Build history of the part. All positions in model axes, mm. Face numbers are marked on the shaded views. A direction names the side the tool comes from. Round coordinates to 2 decimals unless told otherwise and drop trailing zeros. Write each loop counter-clockwise with the first axis right and the second up, starting at its lowest first coordinate (ties: lowest second). Pieces come first, ordered by that corner, then holes. Notation, with made-up numbers: M 87.5,53.25 L 94.5,53.25 A9 ccw 94.5,64.25 Z; hole C -36.5,14 d10. An arc over 180 degrees is marked long. Use a Markdown table: item, result.
from build123d import *

# Parameters (mm, degrees)
F0_W         = 75
F0_H         = 75
F1_DEPTH     = 45
F2_T         = -2.5
F4_T1_DEPTH  = 49.5
F4_T3_DEPTH  = 69
F4_T5_DEPTH  = 69
F4_S9_W      = 3
F4_S9_H      = 3
F4_T10_DEPTH = 3
F4_S15_W     = 3
F4_S15_H     = 3
F4_T16_DEPTH = 3
F4_S21_W     = 3
F4_S21_H     = 3
F4_T22_DEPTH = 3
F4_S27_W     = 3
F4_S27_H     = 3
F4_T28_DEPTH = 3


# Not quite as in the source:
# - a fillet or chamfer that OpenCascade refuses, or shapes differently, is made with other operations: its cross-section is extruded or revolved along the edge and cut away or added
# - a feature of the source that left no trace in its solid (it failed there, or was rolled back) is left out


with BuildPart() as f1:
    # F0 (on Front) → F1 (new body)
    with BuildSketch(Plane.XZ):
        Rectangle(F0_W, F0_H)
    extrude(amount=F1_DEPTH)

    # F2
    f2_openings = [f1.faces().sort_by_distance(p)[0] for p in [
        (0, -45, 0),
    ]]
    offset(amount=F2_T, openings=f2_openings)

    # F4: fillet of radius 3 on 8 edges, made by hand

    # F4_s2 → F4_t1 (cut)
    with BuildSketch(Plane.XZ.offset(-7.5)):
        with BuildLine():
            ThreePointArc((-34.5, 37.5), (-36.6213203436, 36.6213203436), (-37.5, 34.5))
            Line((-37.5, 34.5), (-37.5, 37.5))
            Line((-37.5, 37.5), (-34.5, 37.5))
        make_face()
        with BuildLine():
            ThreePointArc((-34.5, -37.5), (-36.6213203436, -36.6213203436), (-37.5, -34.5))
            Line((-37.5, -34.5), (-37.5, -37.5))
            Line((-37.5, -37.5), (-34.5, -37.5))
        make_face()
        with BuildLine():
            ThreePointArc((34.5, -37.5), (36.6213203436, -36.6213203436), (37.5, -34.5))
            Line((37.5, -34.5), (37.5, -37.5))
            Line((37.5, -37.5), (34.5, -37.5))
        make_face()
        with BuildLine():
            ThreePointArc((37.5, 34.5), (36.6213203436, 36.6213203436), (34.5, 37.5))
            Line((34.5, 37.5), (37.5, 37.5))
            Line((37.5, 37.5), (37.5, 34.5))
        make_face()
    extrude(amount=F4_T1_DEPTH, mode=Mode.SUBTRACT)

    # F4_s4 → F4_t3 (cut)
    with BuildSketch(Plane.YZ.offset(-34.5)):
        with BuildLine():
            ThreePointArc((-42, -37.5), (-44.1213203436, -36.6213203436), (-45, -34.5))
            Line((-45, -34.5), (-45, -37.5))
            Line((-45, -37.5), (-42, -37.5))
        make_face()
        with BuildLine():
            ThreePointArc((-42, 37.5), (-44.1213203436, 36.6213203436), (-45, 34.5))
            Line((-45, 34.5), (-45, 37.5))
            Line((-45, 37.5), (-42, 37.5))
        make_face()
    extrude(amount=F4_T3_DEPTH, mode=Mode.SUBTRACT)

    # F4_s6 → F4_t5 (cut)
    with BuildSketch(Plane.XY.offset(-34.5)):
        with BuildLine():
            ThreePointArc((37.5, -42), (36.6213203436, -44.1213203436), (34.5, -45))
            Line((34.5, -45), (37.5, -45))
            Line((37.5, -45), (37.5, -42))
        make_face()
        with BuildLine():
            ThreePointArc((-37.5, -42), (-36.6213203436, -44.1213203436), (-34.5, -45))
            Line((-34.5, -45), (-37.5, -45))
            Line((-37.5, -45), (-37.5, -42))
        make_face()
    extrude(amount=F4_T5_DEPTH, mode=Mode.SUBTRACT)


with BuildPart() as f4_tool8:
    # F4_s9 → F4_t10 (new body)
    with BuildSketch(Plane.XY.offset(34.5)):
        with Locations((-36, -43.5)):
            Rectangle(F4_S9_W, F4_S9_H)
    extrude(amount=F4_T10_DEPTH)

    # F4_s11 → F4_t12 (revolve, cut)
    with BuildSketch(Plane(origin=(-34.5, -42, 34.5), x_dir=(0.7071067812, 0.7071067812, 0), z_dir=(0.7071067812, -0.7071067812, 0))):
        with BuildLine():
            ThreePointArc((0, -3), (3, 0), (0, 3))
            Line((0, 3), (0, -3))
        make_face()
    revolve(axis=Axis((-34.5, -42, 34.5), (0, 0, 1)), mode=Mode.SUBTRACT)


with BuildPart() as f1_1:
    add(f1.part)

    # F4_t7: cut F4_tool8
    add(f4_tool8.part, mode=Mode.SUBTRACT)


with BuildPart() as f4_tool14:
    # F4_s15 → F4_t16 (new body)
    with BuildSketch(Plane.XY.offset(-34.5)):
        with Locations((-36, -43.5)):
            Rectangle(F4_S15_W, F4_S15_H)
    extrude(amount=-F4_T16_DEPTH)

    # F4_s17 → F4_t18 (revolve, cut)
    with BuildSketch(Plane(origin=(-34.5, -42, -34.5), x_dir=(0.7071067812, 0.7071067812, 0), z_dir=(-0.7071067812, 0.7071067812, 0))):
        with BuildLine():
            ThreePointArc((0, -3), (3, 0), (0, 3))
            Line((0, 3), (0, -3))
        make_face()
    revolve(axis=Axis((-34.5, -42, -34.5), (0, 0, -1)), mode=Mode.SUBTRACT)


with BuildPart() as f1_2:
    add(f1_1.part)

    # F4_t13: cut F4_tool14
    add(f4_tool14.part, mode=Mode.SUBTRACT)


with BuildPart() as f4_tool20:
    # F4_s21 → F4_t22 (new body)
    with BuildSketch(Plane.XY.offset(-34.5)):
        with Locations((36, -43.5)):
            Rectangle(F4_S21_W, F4_S21_H)
    extrude(amount=-F4_T22_DEPTH)

    # F4_s23 → F4_t24 (revolve, cut)
    with BuildSketch(Plane(origin=(34.5, -42, -34.5), x_dir=(-0.7071067812, 0.7071067812, 0), z_dir=(-0.7071067812, -0.7071067812, 0))):
        with BuildLine():
            ThreePointArc((0, -3), (3, 0), (0, 3))
            Line((0, 3), (0, -3))
        make_face()
    revolve(axis=Axis((34.5, -42, -34.5), (0, 0, -1)), mode=Mode.SUBTRACT)


with BuildPart() as f1_3:
    add(f1_2.part)

    # F4_t19: cut F4_tool20
    add(f4_tool20.part, mode=Mode.SUBTRACT)


with BuildPart() as f4_tool26:
    # F4_s27 → F4_t28 (new body)
    with BuildSketch(Plane.YZ.offset(34.5)):
        with Locations((-43.5, 36)):
            Rectangle(F4_S27_W, F4_S27_H)
    extrude(amount=F4_T28_DEPTH)

    # F4_s29 → F4_t30 (revolve, cut)
    with BuildSketch(Plane(origin=(34.5, -42, 34.5), x_dir=(0, 0.7071067812, -0.7071067812), z_dir=(0, -0.7071067812, -0.7071067812))):
        with BuildLine():
            ThreePointArc((0, -3), (3, 0), (0, 3))
            Line((0, 3), (0, -3))
        make_face()
    revolve(axis=Axis((34.5, -42, 34.5), (1, 0, 0)), mode=Mode.SUBTRACT)


with BuildPart() as f1_4:
    add(f1_3.part)

    # F4_t25: cut F4_tool26
    add(f4_tool26.part, mode=Mode.SUBTRACT)


solid = f1_4.part
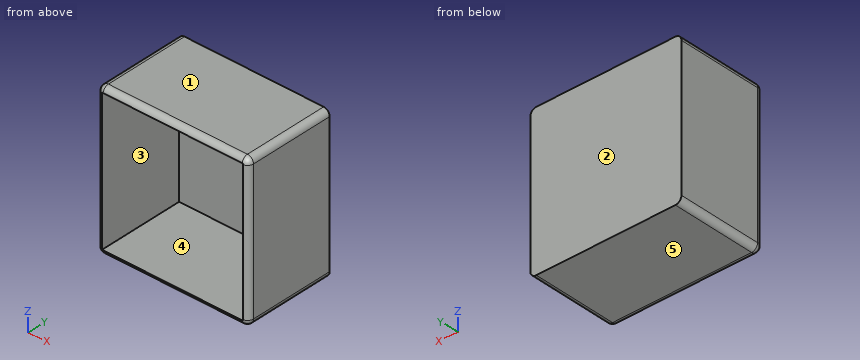
Q1. Cut at A-A on y = -24. Give the cut face in (x, z).
Response values:
| item | result |
|---|---|
| outline | M -37.5,-34.5 A3 ccw -34.5,-37.5 L 34.5,-37.5 A3 ccw 37.5,-34.5 L 37.5,34.5 A3 ccw 34.5,37.5 L -34.5,37.5 A3 ccw -37.5,34.5 Z; hole M -35,-35 L 35,-35 L 35,35 L -35,35 Z |
Q2. Cut at C-C on z = -23.5. Give the cut face in (x, y).
Response values:
| item | result |
|---|---|
| outline | M -37.5,-42 A3 ccw -35,-44.96 L -35,-2.5 L 35,-2.5 L 35,-44.96 A3 ccw 37.5,-42 L 37.5,0 L -37.5,0 Z |
Q3. Two-plate mould, pull along Z, no slides. Class the marked faces 1, 2 and 3: +Z half, -Z half, draft (parallel to the pull), parting line (faces both ways), or undercut.
Response values:
| item | result |
|---|---|
| face 1 | +Z half |
| face 2 | draft |
| face 3 | undercut |
Q4. Cut at B-B on x = -3. Give the cut face in (y, z).
Response values:
| item | result |
|---|---|
| outline | M -44.96,-35 A3 ccw -42,-37.5 L 0,-37.5 L 0,37.5 L -42,37.5 A3 ccw -44.96,35 L -2.5,35 L -2.5,-35 Z |
Q5. Drill centre lines: L1, parallel to Z at x = 12, y = -15; L2, parallel to Y at x = 7, z = -5.5. Where is each one in solid material? Low to high.
Response values:
| item | result |
|---|---|
| L1 | z = -37.5 to -35, 35 to 37.5 |
| L2 | y = -2.5 to 0 |
Q6. Which spindle directions (+Z, -Z, +X, -X, +Y, -Y) get a long thin tool onto all of the face, cutting with end or side? Do the marked faces 4 and 5. Say none if no direction does.
Response values:
| item | result |
|---|---|
| face 4 | -Y |
| face 5 | -Z, +X, -X, +Y, -Y |
